Source: CAD feature listing. Evaluate the final solid. Frame: model axes, mm. A direction names the side the tool comes from. Give positions to 0.01 mm unless a question says otherwise; leave off trailing zeros. Write each loop counter-clockwise with the first axis right and the second up, starting at its lowest first coordinate (ties: lowest second). Pieces come first, ordered by that corner, then holes. Notation, with made-up numbers: (-29.5, 40.25) -> (13.5, 40.25) arc R8 cw to (13.5, 51.25) -> close; hole circle Ø1 at (71, 23.5). An arc over 180 degrees is marked (long way). Use a Markdown table: item, result. Add a question column.
```python
from build123d import *

# Parameters (mm, degrees)
F4_R     = 21
F5_DEPTH = 20
F6_R     = 7.9
F7_DEPTH = 10
F8_R     = 7
F9_DEPTH = 7.3
F10_R    = 0.5


with BuildPart() as f5:
    # F4 (on Top) → F5 (new body)
    with BuildSketch(Plane.XY):
        Circle(F4_R)
    extrude(amount=F5_DEPTH)

    # F6 (on Top) → F7 (cut)
    with BuildSketch(Plane.XY):
        Circle(F6_R)
    extrude(amount=F7_DEPTH, mode=Mode.SUBTRACT)

    # F8 (on face) → F9 (join)
    with BuildSketch(Plane.XY.offset(20)):
        Circle(F8_R)
    extrude(amount=F9_DEPTH)

    # F10
    f10_edges = [f5.edges().sort_by_distance(p)[0] for p in [
        (-7, 0, 27.3),
        (-21, 0, 20),
        (-21, 0, 0),
        (-7.9, 0, 0),
        (-7.9, 0, 10),
    ]]
    fillet(f10_edges, radius=F10_R)


solid = f5.part
```
(1) Mould query, pull axis X, two halves, no side actions, for faces 3 (the flat face through (9, 0, 0)), 4 (the cylindrical face through (6.466, -2.681, 23.352)), 5 (the cylindrical face through (-6.269, -4.807, 4.937)), 6 (the flat face through (0, 0, 10)). Classes: +X half, -X half, draft (parallel to the pull), parting line (faces both ways), or undercut.
(2) Material intervals for L1, parallel to Y at x = 0, z = 5.5; L2, parallel to Z at x = 16.5, y = 0.5; L3, parallel to Z at x = 0.5, y = 6, sorted ascending.
(3) Cut plane C-C on z = 15.5. Return the cut outline in (x, y), then the cut area to 3 significant figures.
(4) Access query for faces 1 (the flat face through (0, 0, 27.3)), 2 (the flat face through (9, 0, 20)). Directions: +Z, -Z, +X, -X, +Y, -Y. A direction counts if a zero-diameter tool reaches every point of the face in a straight line with its end or side. Return the directions, or none.
(5) Cut plane A-A on y = 0. Return the cut outline in (x, z).
(6) First-contact query: pin 1 Ø1 at (x, z) = (10.5, 8) entering from +Y; pin 2 Ø4.5 at (x, y) = (-2.5, 3.5) entering from -Z; pin 3 Ø6 at (x, z) = (-15, 20) entering from +Y. Flat tips, straight axial feed; report the tip coordinate or a pass-through.
(7) Cut plane D-D on z = 22.5. Return the cut outline in (x, y).
Output:
| question | item | result |
|---|---|---|
| 1 | face 3 | draft |
| 1 | face 4 | parting line |
| 1 | face 5 | undercut |
| 1 | face 6 | undercut |
| 2 | L1 | -21 to -7.9, 7.9 to 21 |
| 2 | L2 | 0 to 20 |
| 2 | L3 | 10 to 27.3 |
| 3 | outline | circle Ø42 at (0, 0) |
| 3 | area | 1,390 mm^2 |
| 4 | face 1 | +Z, +X, -X, +Y, -Y |
| 4 | face 2 | +Z |
| 5 | outline | (-21, 0.5) arc R0.5 ccw to (-20.5, 0) -> (-8.4, 0) arc R0.5 ccw to (-7.9, 0.5) -> (-7.9, 9.5) arc R0.5 cw to (-7.4, 10) -> (7.4, 10) arc R0.5 cw to (7.9, 9.5) -> (7.9, 0.5) arc R0.5 ccw to (8.4, 0) -> (20.5, 0) arc R0.5 ccw to (21, 0.5) -> (21, 19.5) arc R0.5 ccw to (20.5, 20) -> (7, 20) -> (7, 26.8) arc R0.5 ccw to (6.5, 27.3) -> (-6.5, 27.3) arc R0.5 ccw to (-7, 26.8) -> (-7, 20) -> (-20.5, 20) arc R0.5 ccw to (-21, 19.5) -> close |
| 6 | pin 1 | y = 18.47 |
| 6 | pin 2 | z = 10 |
| 6 | pin 3 | y = 17.21 |
| 7 | outline | circle Ø14 at (0, 0) |
